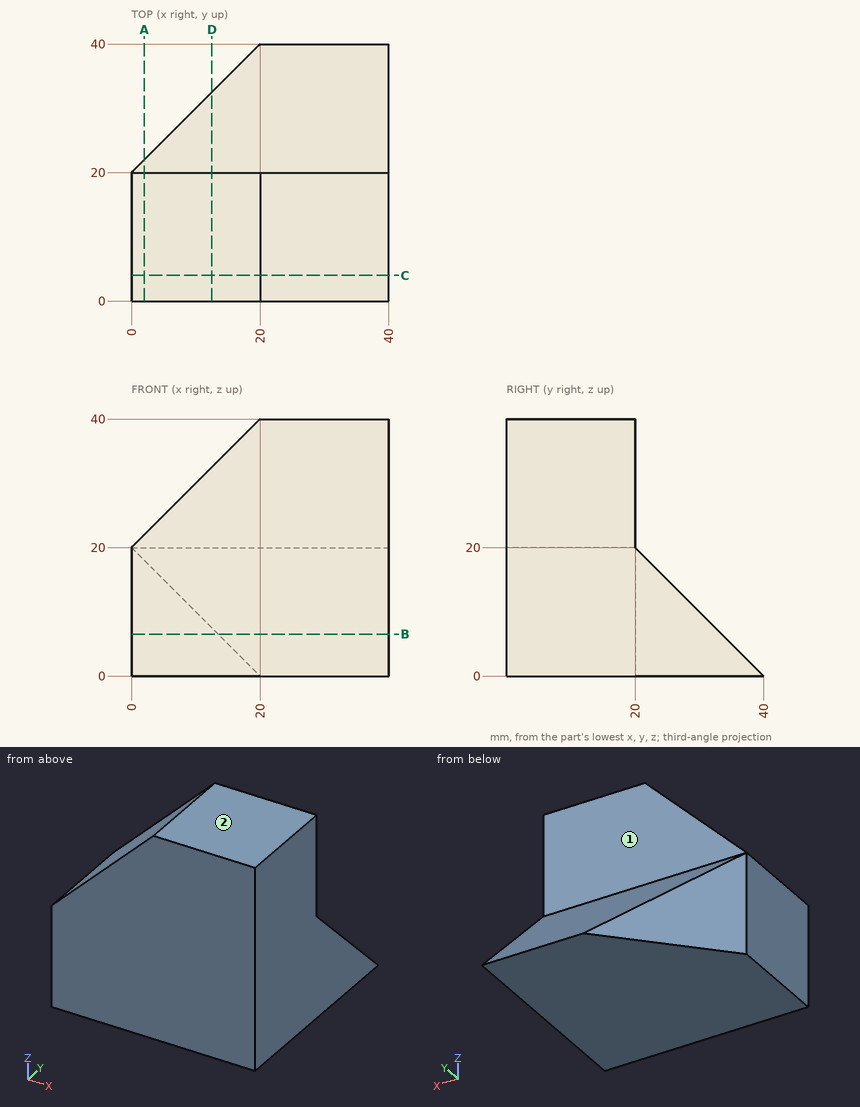
Input: dimensioned drawing with shaded views. Units: mm. Origin: part minimum x, y, z. A direction names the side the tool comes from. Give positions to 0.01 mm unless a question says otherwise; leave off trailing zeros. Loops run counter-clockwise (first coordinate to the right, second up) from the corner with the lowest first, then second, coordinate; pieces in that order, holes last. Notation, with made-up numbers: (11.5, 12) -> (69.5, 12) arc R28 ccw to (69.5, 42) -> close; hole circle Ø5 at (31.25, -22.75). An arc over 180 degrees is marked (long way). Use a Markdown table: item, result. Add a question column.
1) Section query B-B, the plane z = 6.5. Return the cut outline in (x, y).
2) Reachability of the marked faces 1 and 2 from +Z, -Z, +X, -X, +Y, -Y: full face, straight path, thin tool, end or side. Return the list, or none.
3) First-contact query: pin 1 (22 mm diameter, centred on x = 23.5, z = 28.5, fed in from +Y); pin 2 (2 mm diameter, centred on x = 7, z = 10.5, fed in from +Y). Flat tips, straight axial feed; report the tip coordinate or a pass-through.
4) Section query A-A, the plane x = 2. Return the cut outline in (y, z).
5) Section query D-D, the plane x = 12.5. Return the cut outline in (y, z).
6) Section query C-C, the plane y = 4. Return the cut outline in (x, z).
7) Line query: line 1 along Y through (x, z) = (23, 27.5); line 2 along Z through (x, y) = (32, 37.5); line 3 along Z through (x, y) = (21, 33.5). Output: solid intervals per line, ascending. Write a range as [from, to].
Numbers:
| question | item | result |
|---|---|---|
| 1 | outline | (0, 0) -> (40, 0) -> (40, 33.5) -> (13.5, 33.5) -> (0, 20) -> close |
| 2 | face 1 | +Z, +X, -X, +Y |
| 2 | face 2 | +Z, +X, -X, +Y, -Y |
| 3 | pin 1 | stops at y = 22.5 |
| 3 | pin 2 | stops at y = 28 |
| 4 | outline | (0, 0) -> (22, 0) -> (22, 18) -> (20, 20) -> (20, 22) -> (0, 22) -> close |
| 5 | outline | (0, 0) -> (32.5, 0) -> (32.5, 7.5) -> (20, 20) -> (20, 32.5) -> (0, 32.5) -> close |
| 6 | outline | (0, 0) -> (40, 0) -> (40, 40) -> (20, 40) -> (0, 20) -> close |
| 7 | line 1 | y = [0, 20] |
| 7 | line 2 | z = [0, 2.5] |
| 7 | line 3 | z = [0, 6.5] |
